Geometry check sheet. Reference: the model listing, model coordinates, mm. A direction names the side the tool comes from. Round coordinates to 2 decimals unless told otherwise and drop trailing zeros. Order: outer loops, then holes, each group sorted by start corner. A loop starts at its lowest first (then second) coordinate and runs counter-clockwise, first axis right, second up.
(1) Cross-section at C-C on y = 11. Enter the section's corners in (x, z).
(2) Thickness scan on L1, parallel to Z at x = 0, y = 10.75; L2, parallel to Y at x = -55.5, z = -85; L3, parallel to Z at x = -26, y = 9.5. Record the ranges inside material, lowest first.
(3) Set-up check for faces 1 (the face through (16, 1, 100)), 2 (the face through (1, 17, -21)): record each of +Z, -Z, +X, -X, +Y, -Y from which the full face is reachable in a straight line by a thin tool's end or side.
(4) Cross-section at D-D on x = -57.5. Enter the section's corners in (y, z), and give its area (3 significant figures).
(5) Gauge pin test, flat ends, axial feed: P1, Ø3, axis at x = 81, y = 3, coming from the -Z side; P2, Ø2, axis at x = 44.5, y = 7, coming from the +Z side; P3, Ø1, axis at y = 5, z = -52.5, coming from the +X side. Record the tip position at first contact, or that the pin passes through.
(6) Cross-section at B-B on x = 0. Enter the section's corners in (y, z), and give its area (3 significant figures).
(7) Draft check along Z on faces 3 (the face through (16, 16, 100)), 4 (the face through (2.17, 8.38, 9.76)), 5 (the face through (22.33, 16.51, -100.55)). Enter one of: pulls with the +Z half, pulls with the -Z half, needs draft (parallel to the pull), parting line crosses it, or undercut.
(8) Cross-section at A-A on z = 0. Enter the section's corners in (x, y).
Autodesk Inventor part; units mm, degrees
ref_plane "YZ Plane" through (0, 0, 0) normal (1, 0, 0) x (0, 1, 0)
ref_plane "XZ Plane" through (0, 0, 0) normal (0, 1, 0) x (-1, 0, 0)
ref_plane "XY Plane" through (0, 0, 0) normal (0, 0, 1) x (1, 0, 0)
sketch "Sketch1" plane through (0, 0, 0) normal (0, 0, 1) x (1, 0, 0)
  line L0 (0, 0) -> (-103, 0)
  line L1 (-103, 0) -> (-103, 1)
  line L2 (-103, 1) -> (-100, 1)
  line L3 (-100, 1) -> (-100, 16)
  line L4 (-100, 16) -> (-103, 16)
  line L5 (-103, 16) -> (-103, 17)
  line L6 (-103, 17) -> (-10, 17)
  line L7 (-10, 17) -> (-10, 0)
  line L8 (0, 0) -> (0, 15.4715) construction
  dimension "d0" = 100
  dimension "d1" = 15
  dimension "d2" = 1
  dimension "d3" = 1
  dimension "d4" = 10
  dimension "d5" = 3
revolve "Revolution1" add sketch "Sketch1" angle 360 about axis through (0, 0, 0) along (0, 1, 0)
properties part number "fakepully"
Found:
1. outline: circle Ø200 at (0, 0); hole circle Ø20 at (0, 0)
2. L1: z = -100 to -10, 10 to 100
2. L2: y = 0 to 1, 16 to 17
2. L3: z = -96.56 to 96.56
3. face 1: none
3. face 2: +Z, -Z, +X, -X, +Y
4. outline: (0, -85.46) - (1, -85.46) - (1, -81.82) - (16, -81.82) - (16, -85.46) - (17, -85.46) - (17, 85.46) - (16, 85.46) - (16, 81.82) - (1, 81.82) - (1, 85.46) - (0, 85.46) - close
4. area: 2,800 mm2
5. P1: stops at z = -60.66
5. P2: stops at z = 90.04
5. P3: stops at x = 85.42
6. outline: (0, -103) - (1, -103) - (1, -100) - (16, -100) - (16, -103) - (17, -103) - (17, -10) - (0, -10) - close; (0, 10) - (17, 10) - (17, 103) - (16, 103) - (16, 100) - (1, 100) - (1, 103) - (0, 103) - close
6. area: 3,070 mm2
7. face 3: needs draft
7. face 4: undercut
7. face 5: parting line crosses it
8. outline: (-103, 0) - (-10, 0) - (-10, 17) - (-103, 17) - (-103, 16) - (-100, 16) - (-100, 1) - (-103, 1) - close; (10, 0) - (103, 0) - (103, 1) - (100, 1) - (100, 16) - (103, 16) - (103, 17) - (10, 17) - close
